```python
from build123d import *

# Parameters (mm, degrees)
SALIENTE_EXTRUIR1_DEPTH                              = 3
SALIENTE_EXTRUIR2_START                              = -3
SALIENTE_EXTRUIR2_DEPTH                              = 3
SALIENTE_EXTRUIR4_DEPTH                              = 3
SALIENTE_EXTRUIR5_DEPTH                              = 50
AVELLANADO_PARA_TORNILLO_CON_CABEZA_PLAN_D           = 2.4
AVELLANADO_PARA_TORNILLO_CON_CABEZA_PLAN_CSINK_D     = 4.4
AVELLANADO_PARA_TORNILLO_CON_CABEZA_PLAN_CSINK_ANGLE = 90
CROQUIS11_R                                          = 2
CORTAR_EXTRUIR2_DEPTH                                = 6
CHAFL_N2_SIZE                                        = 0.3


with BuildPart() as part:
    # Croquis1 → Saliente-Extruir1 (new body)
    with BuildSketch(Plane(origin=(0, 81, 0), x_dir=(1, 0, 0), z_dir=(0, 1, 0))):
        with BuildLine():
            Line((164.5, -35), (164.5, -58))
            Line((164.5, -58), (164.5, -95))
            ThreePointArc((164.5, -95), (162.889087297, -98.889087297), (159, -100.5))
            Line((159, -100.5), (29, -100.5))
            ThreePointArc((29, -100.5), (25.110912703, -98.889087297), (23.5, -95))
            Line((23.5, -95), (23.5, 95))
            ThreePointArc((23.5, 95), (25.110912703, 98.889087297), (29, 100.5))
            Line((29, 100.5), (159, 100.5))
            ThreePointArc((159, 100.5), (162.889087297, 98.889087297), (164.5, 95))
            Line((164.5, 95), (164.5, -35))
        make_face()
    extrude(amount=SALIENTE_EXTRUIR1_DEPTH)

    # Croquis2 → Saliente-Extruir2 (add)
    with BuildSketch(Plane(origin=(0, 81, 0), x_dir=(1, 0, 0), z_dir=(0, 1, 0)).offset(SALIENTE_EXTRUIR2_START)):
        with BuildLine():
            Line((164.5, -95), (164.5, 95))
            ThreePointArc((164.5, 95), (162.889087297, 98.889087297), (159, 100.5))
            Line((159, 100.5), (29, 100.5))
            ThreePointArc((29, 100.5), (25.110912703, 98.889087297), (23.5, 95))
            Line((23.5, 95), (23.5, -95))
            ThreePointArc((23.5, -95), (25.110912703, -98.889087297), (29, -100.5))
            Line((29, -100.5), (159, -100.5))
            ThreePointArc((159, -100.5), (162.889087297, -98.889087297), (164.5, -95))
        make_face()
        with BuildLine():
            Line((162.5, -95), (162.5, 95))
            ThreePointArc((162.5, 95), (161.474873734, 97.474873734), (159, 98.5))
            Line((159, 98.5), (29, 98.5))
            ThreePointArc((29, 98.5), (26.525126266, 97.474873734), (25.5, 95))
            Line((25.5, 95), (25.5, -95))
            ThreePointArc((25.5, -95), (26.525126266, -97.474873734), (29, -98.5))
            Line((29, -98.5), (159, -98.5))
            ThreePointArc((159, -98.5), (161.474873734, -97.474873734), (162.5, -95))
        make_face(mode=Mode.SUBTRACT)
    extrude(amount=SALIENTE_EXTRUIR2_DEPTH)

    # Croquis4 → Saliente-Extruir4 (add)
    with BuildSketch(Plane.XZ.offset(-81)):
        with BuildLine():
            Line((33, -92.5), (155, -92.5))
            ThreePointArc((155, -92.5), (156.060660172, -92.060660172), (156.5, -91))
            Line((156.5, -91), (156.5, 35))
            Line((156.5, 35), (156.5, 58))
            Line((156.5, 58), (156.5, 91))
            ThreePointArc((156.5, 91), (156.060660172, 92.060660172), (155, 92.5))
            Line((155, 92.5), (33, 92.5))
            ThreePointArc((33, 92.5), (31.939339828, 92.060660172), (31.5, 91))
            Line((31.5, 91), (31.5, -91))
            ThreePointArc((31.5, -91), (31.939339828, -92.060660172), (33, -92.5))
        make_face()
        Polygon((33.5, -90.5), (154.5, -90.5), (154.5, 35), (154.5, 58), (154.5, 90.5), (33.5, 90.5), align=None, mode=Mode.SUBTRACT)
    extrude(amount=SALIENTE_EXTRUIR4_DEPTH)

    # Croquis5 → Saliente-Extruir5 (add)
    with BuildSketch(Plane.XZ.offset(-81)):
        with BuildLine():
            Line((155, 92.5), (146.5, 92.5))
            Line((146.5, 92.5), (146.5, 82.5))
            Line((146.5, 82.5), (156.5, 82.5))
            Line((156.5, 82.5), (156.5, 91))
            ThreePointArc((156.5, 91), (156.060660172, 92.060660172), (155, 92.5))
        make_face()
        with BuildLine():
            Line((31.5, -91), (31.5, -82.5))
            Line((31.5, -82.5), (41.5, -82.5))
            Line((41.5, -82.5), (41.5, -92.5))
            Line((41.5, -92.5), (33, -92.5))
            ThreePointArc((33, -92.5), (31.939339828, -92.060660172), (31.5, -91))
        make_face()
    extrude(amount=SALIENTE_EXTRUIR5_DEPTH)

    # Avellanado para tornillo con cabeza plana de M21 (through all)
    with Locations(Plane(origin=(0, 84, 0), x_dir=(1, 0, 0), z_dir=(0, 1, 0))):
        with Locations((138, -13.5), (101, -13.5), (138, -79.5), (101, -79.5)):
            CounterSinkHole(AVELLANADO_PARA_TORNILLO_CON_CABEZA_PLAN_D / 2, AVELLANADO_PARA_TORNILLO_CON_CABEZA_PLAN_CSINK_D / 2, counter_sink_angle=AVELLANADO_PARA_TORNILLO_CON_CABEZA_PLAN_CSINK_ANGLE)

    # Croquis11 → Cortar-Extruir2 (cut)
    with BuildSketch(Plane.XZ.offset(-31)):
        with Locations(Location((36.5, -87.5, 0), (0, 0, 270))):
            Circle(CROQUIS11_R)
        with Locations(Location((151.5, 87.5, 0), (0, 0, 270))):
            Circle(CROQUIS11_R)
    extrude(amount=-CORTAR_EXTRUIR2_DEPTH, mode=Mode.SUBTRACT)

    # Chaflán2
    chafl_n2_edges = [part.edges().sort_by_distance(p)[0] for p in [
        (36.5, 31, -85.5),
        (151.5, 31, 89.5),
    ]]
    chamfer(chafl_n2_edges, length=CHAFL_N2_SIZE)


solid = part.part
```
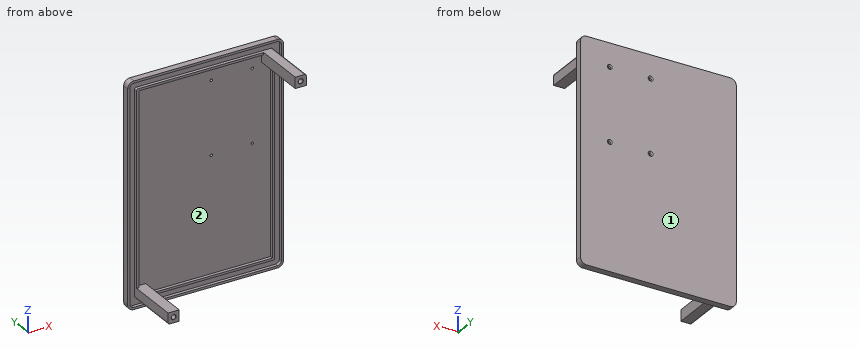
For this review, take the finished solid that the model builds, in its own axes (mm). Face numbers are marked on the shaded views. Give positions to 0.01 mm unless a question says otherwise; leave off trailing zeros. Write each loop counter-clockwise with the first axis right and the second up, starting at its lowest first coordinate (ties: lowest second). Pieces come first, ordered by that corner, then holes.
Item 1: Take a section at A-A (y = 44). Give the boundary of the cut face in (x, z), and give its area (3 significant figures).
Item 2: Take a section at B-B (x = 132.5). Give the boundary of the cut face in (y, z).
Item 3: The part is to be moulded in two halves that separate along Z. For the marked faces 1 and 2, say which applies: +Z half, -Z half, draft (parallel to the pull), parting line (faces both ways), or undercut.
Item 4: Take a section at C-C (z = -74). Give the boundary of the cut face in (x, y).
Item 5: Wall thickness on probe 1 along X at (y, z) = (82, 13.5); probe 2 along Z at (x, y) = (138, 82.6); probe 3 along Y at (x, z) = (123, 69): over which ranges is each line inside the solid? List them lowest first.
Item 6: Insertion check: P1, Ø5, axis at x = 151, y = 53, coming from the -Z side; P2, Ø4, axis at x = 69, z = -42.5, coming from the -Y side; P3, Ø3, axis at x = 37, z = -88, coming from the -Y side; P4, Ø12, axis at x = 140, y = 39.5, coming from the +Z side. Each pin has a flat end and moves straight along its axis. Give the tip position at first contact, or say it passes through.
Established:
1. outline: (31.5, -91) arc R1.5 ccw to (33, -92.5) - (41.5, -92.5) - (41.5, -82.5) - (31.5, -82.5) - close; (146.5, 82.5) - (156.5, 82.5) - (156.5, 91) arc R1.5 ccw to (155, 92.5) - (146.5, 92.5) - close
1. area: 199 mm2
2. outline: (78, -100.5) - (84, -100.5) - (84, 100.5) - (78, 100.5) - (78, 98.5) - (81, 98.5) - (81, 92.5) - (78, 92.5) - (78, 90.5) - (81, 90.5) - (81, -90.5) - (78, -90.5) - (78, -92.5) - (81, -92.5) - (81, -98.5) - (78, -98.5) - close
3. face 1: draft
3. face 2: undercut
4. outline: (23.5, 78) - (25.5, 78) - (25.5, 81) - (31.5, 81) - (31.5, 78) - (33.5, 78) - (33.5, 81) - (154.5, 81) - (154.5, 78) - (156.5, 78) - (156.5, 81) - (162.5, 81) - (162.5, 78) - (164.5, 78) - (164.5, 84) - (23.5, 84) - close
5. probe 1: x = 23.5 to 99.8, 102.2 to 136.8, 139.2 to 164.5
5. probe 2: z = -100.5 to 12.3, 14.7 to 78.3, 80.7 to 100.5
5. probe 3: y = 81 to 84
6. P1: stops at z = 82.5
6. P2: stops at y = 81
6. P3: stops at y = 31.09
6. P4: passes through
